Read the model definition and answer for the solid it produces. Units are mm, in the model's axes. Coordinates: 2 decimals unless noted, no trailing zeros. Loops run counter-clockwise (first coordinate to the right, second up) from the corner with the lowest first, then second, coordinate; pieces in that order, holes last. Notation, with made-up numbers: (89, 65.25) - (136, 65.25) arc R17 cw to (136, 72.25) - close; hole circle Ø11 at (55.5, -17). An arc over 180 degrees is marked (long way). Use one line per item in the form item = value.
from build123d import *

# Parameters (mm, degrees)
SKETCH1_W           = 200
SKETCH1_H           = 200
SKETCH1_R           = 10
BOSS_EXTRUDE1_DEPTH = 30
BOSS_EXTRUDE2_START = -10
SKETCH2_R           = 10
BOSS_EXTRUDE2_DEPTH = 20


with BuildPart() as part:
    # Sketch1 → Boss-Extrude1 (new body)
    with BuildSketch(Plane.XY):
        with Locations((100, 100)):
            Rectangle(SKETCH1_W, SKETCH1_H)
        with Locations((145, 130)):
            Circle(SKETCH1_R, mode=Mode.SUBTRACT)
        with Locations((55, 130)):
            Circle(SKETCH1_R, mode=Mode.SUBTRACT)
    extrude(amount=BOSS_EXTRUDE1_DEPTH)

    # Sketch2 → Boss-Extrude2 (add)
    with BuildSketch(Plane(origin=(0, 0, 0), x_dir=(-1, 0, 0), z_dir=(0, 0, -1)).offset(BOSS_EXTRUDE2_START)):
        with Locations((-145, 130)):
            Circle(SKETCH2_R)
        with Locations((-55, 130)):
            Circle(SKETCH2_R)
    extrude(amount=-BOSS_EXTRUDE2_DEPTH)


solid = part.part
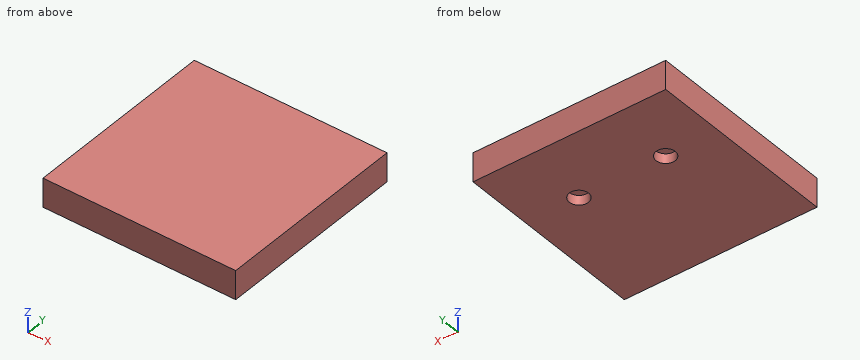
Item 1: The part is cut by section B-B on z = 6. Give the vertices of the cut face in (x, y), plus the area to 3 significant figures.
Results below:
outline = (0, 0) - (200, 0) - (200, 200) - (0, 200) - close; hole circle Ø20 at (55, 130); hole circle Ø20 at (145, 130)
area = 39,400 mm²
Item 2: The part is cut by section A-A on y = 130. Give the vertices of the cut face in (x, z), plus the area to 3 significant figures.
Results below:
outline = (0, 0) - (45, 0) - (45, 10) - (65, 10) - (65, 0) - (135, 0) - (135, 10) - (155, 10) - (155, 0) - (200, 0) - (200, 30) - (0, 30) - close
area = 5,600 mm²
Item 3: Find the intervals of material crossed by L1, parallel to Y at x = 145, z = 7; L2, parallel to Y at x = 151, z = 9.75, in increasing order.
Results below:
L1 = 0 to 120, 140 to 200
L2 = 0 to 122, 138 to 200
Item 4: The part is cut by section C-C on x = 145. Give the vertices of the cut face in (y, z), plus the area to 3 significant figures.
Results below:
outline = (0, 0) - (120, 0) - (120, 10) - (140, 10) - (140, 0) - (200, 0) - (200, 30) - (0, 30) - close
area = 5,800 mm²
Item 5: Each of these flat-tipped pins is pushed along its axis until it touches: P1, Ø1.5, axis at y = 172, z = 6, coming from the -X side; P2, Ø16, axis at x = 54.5, y = 128.5, coming from the -Z side. Where does it stop, or does it pass through?
Results below:
P1 = 0
P2 = 10
